```python
from build123d import *

# Parameters (mm, degrees)
SKETCH2_W           = 110
SKETCH2_H           = 110
BOSS_EXTRUDE1_DEPTH = 100
SKETCH3_W           = 104
SKETCH3_H           = 94
CUT_EXTRUDE1_DEPTH  = 107
SKETCH4_W           = 80
SKETCH4_H           = 60
CUT_EXTRUDE2_DEPTH  = 10
SKETCH5_W           = 20
SKETCH5_H           = 6
BOSS_EXTRUDE2_DEPTH = 107
SKETCH6_W           = 5
SKETCH6_H           = 2
CUT_EXTRUDE3_DEPTH  = 107
SKETCH7_W           = 25
SKETCH7_H           = 6
SKETCH7_W_2         = 5
BOSS_EXTRUDE3_DEPTH = 107
SKETCH8_W           = 5
SKETCH8_H           = 2
CUT_EXTRUDE4_DEPTH  = 107
SKETCH9_W           = 10
SKETCH9_H           = 10
BOSS_EXTRUDE4_DEPTH = 110
SKETCH11_W          = 7
SKETCH11_H          = 7
CUT_EXTRUDE5_DEPTH  = 90
SKETCH13_R          = 1.5
CUT_EXTRUDE6_DEPTH  = 19


with BuildPart() as part:
    # Sketch2 → Boss-Extrude1 (new body)
    with BuildSketch(Plane(origin=(0, 0, 0), x_dir=(1, 0, 0), z_dir=(0, 1, 0))):
        with Locations((55, 55)):
            Rectangle(SKETCH2_W, SKETCH2_H)
    extrude(amount=BOSS_EXTRUDE1_DEPTH)

    # Sketch3 → Cut-Extrude1 (cut)
    with BuildSketch(Plane.ZY):
        with Locations((-55, 50)):
            Rectangle(SKETCH3_W, SKETCH3_H)
    extrude(amount=-CUT_EXTRUDE1_DEPTH, mode=Mode.SUBTRACT)

    # Sketch4 → Cut-Extrude2 (cut)
    with BuildSketch(Plane(origin=(0, 100, 0), x_dir=(1, 0, 0), z_dir=(0, 1, 0))):
        with Locations((40, 55)):
            Rectangle(SKETCH4_W, SKETCH4_H)
    extrude(amount=-CUT_EXTRUDE2_DEPTH, mode=Mode.SUBTRACT)

    # Sketch5 → Boss-Extrude2 (add)
    with BuildSketch(Plane.ZY.offset(-107)):
        with Locations((-97, 89)):
            Rectangle(SKETCH5_W, SKETCH5_H)
        with Locations((-13, 89)):
            Rectangle(SKETCH5_W, SKETCH5_H)
    extrude(amount=BOSS_EXTRUDE2_DEPTH)

    # Sketch6 → Cut-Extrude3 (cut)
    with BuildSketch(Plane.ZY):
        with Locations((-89.5, 89)):
            Rectangle(SKETCH6_W, SKETCH6_H)
        with Locations((-20.5, 89)):
            Rectangle(SKETCH6_W, SKETCH6_H)
    extrude(amount=-CUT_EXTRUDE3_DEPTH, mode=Mode.SUBTRACT)

    # Sketch7 → Boss-Extrude3 (add)
    with BuildSketch(Plane.ZY.offset(-107)):
        with Locations((-94.5, 11)):
            Rectangle(SKETCH7_W, SKETCH7_H)
        with Locations((-15.5, 11)):
            Rectangle(SKETCH7_W, SKETCH7_H)
        with Locations((-104.5, 46)):
            Rectangle(SKETCH7_W_2, SKETCH7_H)
        with Locations((-5.5, 46)):
            Rectangle(SKETCH7_W_2, SKETCH7_H)
    extrude(amount=BOSS_EXTRUDE3_DEPTH)

    # Sketch8 → Cut-Extrude4 (cut)
    with BuildSketch(Plane.ZY):
        with Locations((-5.5, 46)):
            Rectangle(SKETCH8_W, SKETCH8_H)
        with Locations((-84.5, 11)):
            Rectangle(SKETCH8_W, SKETCH8_H)
        with Locations((-25.5, 11)):
            Rectangle(SKETCH8_W, SKETCH8_H)
        with Locations((-104.5, 46)):
            Rectangle(SKETCH8_W, SKETCH8_H)
    extrude(amount=-CUT_EXTRUDE4_DEPTH, mode=Mode.SUBTRACT)

    # Sketch9 → Boss-Extrude4 (add)
    with BuildSketch(Plane(origin=(110, 0, 0), x_dir=(0, 0, -1), z_dir=(1, 0, 0))):
        with Locations((5, 5)):
            Rectangle(SKETCH9_W, SKETCH9_H)
        with Locations((105, 5)):
            Rectangle(SKETCH9_W, SKETCH9_H)
        with Locations((105, 95)):
            Rectangle(SKETCH9_W, SKETCH9_H)
        with Locations((5, 95)):
            Rectangle(SKETCH9_W, SKETCH9_H)
    extrude(amount=-BOSS_EXTRUDE4_DEPTH)

    # Sketch11 → Cut-Extrude5 (cut)
    with BuildSketch(Plane(origin=(110, 0, 0), x_dir=(0, 0, -1), z_dir=(1, 0, 0))):
        with Locations((3.5, 96.5)):
            Rectangle(SKETCH11_W, SKETCH11_H)
        with Locations((106.5, 96.5)):
            Rectangle(SKETCH11_W, SKETCH11_H)
        with Locations((3.5, 3.5)):
            Rectangle(SKETCH11_W, SKETCH11_H)
        with Locations((106.5, 3.5)):
            Rectangle(SKETCH11_W, SKETCH11_H)
    extrude(amount=-CUT_EXTRUDE5_DEPTH, mode=Mode.SUBTRACT)

    # Sketch13 → Cut-Extrude6 (cut)
    with BuildSketch(Plane.ZY):
        with Locations((-106.5, 3.5)):
            Circle(SKETCH13_R)
        with Locations((-3.5, 96.5)):
            Circle(SKETCH13_R)
        with Locations((-106.5, 96.5)):
            Circle(SKETCH13_R)
        with Locations((-3.5, 3.5)):
            Circle(SKETCH13_R)
    extrude(amount=-CUT_EXTRUDE6_DEPTH, mode=Mode.SUBTRACT)


solid = part.part
```
Verification items for the finished model (mm, model axes). A direction names the side the tool comes from. Coordinates: 2 decimals unless noted, no trailing zeros. Write each loop counter-clockwise with the first axis right and the second up, starting at its lowest first coordinate (ties: lowest second). Pieces come first, ordered by that corner, then holes. Notation, with made-up numbers: (80, 32) - (107, 32) arc R22 ccw to (107, 57) - close; hole circle Ø10 at (-10.5, 52). An arc over 180 degrees is marked (long way). One line per question, with ' | ' between items. Start each with the question number.
1. Draft check along Z on faces 4 (the flat face through (54, 49, 0)), 5 (the flat face through (39, 99, -85)), 6 (the flat face through (66, 7, -3)). Enter one of: released by +Z, released by -Z, zero draft, split by the parting line, or undercut.
2. Gauge pin test, flat ends, axial feed: P1, Ø4, axis at y = 39.5, z = -45, coming from the -X side; P2, Ø5.5, axis at x = 64.5, z = -108, coming from the -Y side; P3, Ø3.5, axis at y = 96.5, z = -3.5, coming from the +X side. Record the tip position at first contact, or that the pin passes through.
3. Material ranges on line 1 along Y through (x, z) = (47.5, -5); line 2 along Y through (x, z) = (105.5, -12); line 3 along Y through (x, z) = (61.5, -83), recorded low to high.
4. Section check B-B (y = 78). Enter the section's corners in (x, z), plus the area to 3 significant figures.
5. Section check A-A (z = -20). Enter the section's corners in (x, y), plus the area to 3 significant figures.
6. Section check D-D (z = -71.5). Enter the section's corners in (x, y), plus the area to 3 significant figures.
7. Section check C-C (x = 13). Count the separate pieces of the cut face and the enclosed holes in it, plus the area to 3 significant figures.
8. Access from +Z, -Z, +X, -X, +Y, -Y to the whole of each face (thin tool, end or side, straight path). Record for faces 1 (the flat face through (53, 88, -90)), 2 (the flat face through (110, 49, -54)), 3 (the flat face through (66, 93, -3)).
Computed values:
1) face 4: released by +Z | face 5: undercut | face 6: zero draft
2) P1: x = 107 | P2: y = 7 | P3: x = 20
3) line 1: 7 to 14, 43 to 45, 47 to 49, 86 to 93 | line 2: 0 to 3, 8 to 14, 86 to 92, 97 to 100 | line 3: 0 to 3, 8 to 10, 12 to 14
4) outline: (0, -110) - (110, -110) - (110, 0) - (0, 0) - (0, -3) - (107, -3) - (107, -107) - (0, -107) - close | area: 972 mm²
5) outline: (0, 0) - (110, 0) - (110, 100) - (0, 100) - (0, 97) - (107, 97) - (107, 92) - (0, 92) - (0, 90) - (107, 90) - (107, 88) - (0, 88) - (0, 86) - (107, 86) - (107, 14) - (0, 14) - (0, 8) - (107, 8) - (107, 3) - (0, 3) - close | area: 2,010 mm²
6) outline: (0, 0) - (110, 0) - (110, 100) - (80, 100) - (80, 97) - (107, 97) - (107, 3) - (0, 3) - close | area: 702 mm²
7) separate pieces: 1 | enclosed holes: 4 | area: 1,700 mm²
8) face 1: -X | face 2: +Z, -Z, +X, +Y, -Y | face 3: +Z, +X, +Y
